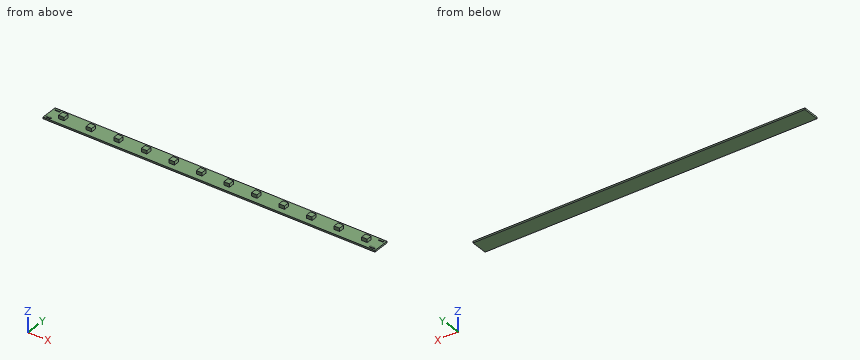
```python
from build123d import *

# Parameters (mm, degrees)
F0_W     = 200
F0_H     = 10
F1_DEPTH = 1
F2_W     = 3.3
F2_H     = 3.3
F3_DEPTH = 2
F5_DEPTH = 0.3


with BuildPart() as f1:
    # F0 (on Top) → F1 (new body)
    with BuildSketch(Plane.XY):
        with Locations((100, 5)):
            Rectangle(F0_W, F0_H)
    extrude(amount=F1_DEPTH)

    # F2 (on face) → F3 (join)
    with BuildSketch(Plane.XY.offset(1)):
        with Locations((8.65, 5)):
            Rectangle(F2_W, F2_H)
        with Locations((25.25, 5)):
            Rectangle(F2_W, F2_H)
        with Locations((41.85, 5)):
            Rectangle(F2_W, F2_H)
        with Locations((58.45, 5)):
            Rectangle(F2_W, F2_H)
        with Locations((75.05, 5)):
            Rectangle(F2_W, F2_H)
        with Locations((91.65, 5)):
            Rectangle(F2_W, F2_H)
        with Locations((108.25, 5)):
            Rectangle(F2_W, F2_H)
        with Locations((124.85, 5)):
            Rectangle(F2_W, F2_H)
        with Locations((141.45, 5)):
            Rectangle(F2_W, F2_H)
        with Locations((158.05, 5)):
            Rectangle(F2_W, F2_H)
        with Locations((174.65, 5)):
            Rectangle(F2_W, F2_H)
        with Locations((191.25, 5)):
            Rectangle(F2_W, F2_H)
    extrude(amount=F3_DEPTH)

    # F4 (on face) → F5 (join)
    with BuildSketch(Plane.XY.offset(1)):
        with BuildLine():
            ThreePointArc((1.001016, 1.177174), (1.088884, 0.965042), (1.301016, 0.877174))
            Line((1.301016, 0.877174), (3.701016, 0.877174))
            ThreePointArc((3.701016, 0.877174), (3.913148, 0.965042), (4.001016, 1.177174))
            Line((4.001016, 1.177174), (4.001016, 1.456027))
            ThreePointArc((4.001016, 1.456027), (3.913148, 1.668159), (3.701016, 1.756027))
            Line((3.701016, 1.756027), (1.301016, 1.756027))
            ThreePointArc((1.301016, 1.756027), (1.088884, 1.668159), (1.001016, 1.456027))
            Line((1.001016, 1.456027), (1.001016, 1.177174))
        make_face()
        with BuildLine():
            ThreePointArc((198.629966, 8.232874), (198.842098, 8.320742), (198.929966, 8.532874))
            Line((198.929966, 8.532874), (198.929966, 8.811727))
            ThreePointArc((198.929966, 8.811727), (198.842098, 9.023859), (198.629966, 9.111727))
            Line((198.629966, 9.111727), (196.229966, 9.111727))
            ThreePointArc((196.229966, 9.111727), (196.017834, 9.023859), (195.929966, 8.811727))
            Line((195.929966, 8.811727), (195.929966, 8.532874))
            ThreePointArc((195.929966, 8.532874), (196.017834, 8.320742), (196.229966, 8.232874))
            Line((196.229966, 8.232874), (198.629966, 8.232874))
        make_face()
        with BuildLine():
            ThreePointArc((198.629966, 0.877174), (198.842098, 0.965042), (198.929966, 1.177174))
            Line((198.929966, 1.177174), (198.929966, 1.456027))
            ThreePointArc((198.929966, 1.456027), (198.842098, 1.668159), (198.629966, 1.756027))
            Line((198.629966, 1.756027), (196.229966, 1.756027))
            ThreePointArc((196.229966, 1.756027), (196.017834, 1.668159), (195.929966, 1.456027))
            Line((195.929966, 1.456027), (195.929966, 1.277174))
            ThreePointArc((195.929966, 1.277174), (196.047123, 0.994331), (196.329966, 0.877174))
            Line((196.329966, 0.877174), (198.629966, 0.877174))
        make_face()
        with BuildLine():
            ThreePointArc((3.701016, 8.232874), (3.913148, 8.320742), (4.001016, 8.532874))
            Line((4.001016, 8.532874), (4.001016, 8.811727))
            ThreePointArc((4.001016, 8.811727), (3.913148, 9.023859), (3.701016, 9.111727))
            Line((3.701016, 9.111727), (1.301016, 9.111727))
            ThreePointArc((1.301016, 9.111727), (1.088884, 9.023859), (1.001016, 8.811727))
            Line((1.001016, 8.811727), (1.001016, 8.532874))
            ThreePointArc((1.001016, 8.532874), (1.088884, 8.320742), (1.301016, 8.232874))
            Line((1.301016, 8.232874), (3.701016, 8.232874))
        make_face()
    extrude(amount=F5_DEPTH)


solid = f1.part
```
For this review, take the finished solid that the model builds, in its own axes (mm). Coordinates: 2 decimals unless noted, no trailing zeros. Write each loop counter-clockwise with the first axis right and the second up, starting at its lowest first coordinate (ties: lowest second). Pieces come first, ordered by that corner, then holes. Notation, with made-up numbers: (15.5, 35.5) - (57.5, 35.5) arc R26 cw to (57.5, 54.5) - close; hole circle Ø10 at (-31, 66.5). An arc over 180 degrees is marked (long way). Answer in a Markdown table with one row per item. Add a question column.
Q1. We need section B-B, the plane x = 152.5. State the section outline as (y, z) points, and give its area (3 significant figures).
Q2. For P1, Ø1, axis at y = 5, z = 2, coming from the +X side; P2, Ø2, axis at x = 49.5, y = 9, coming from the +Z side; P3, Ø1, axis at x = 8.5, z = 2.5, coming from the -Y side, all flat-tipped, find the tip position at first contact; note any pin that passes through.
Q3. For probe 1 along Z at (x, y) = (161, 4.75); probe 2 along Y at (x, z) = (57.5, 2.6), list the stretches that pass through material, from the lowest coordinate up.
Q4. We need section A-A, the plane z = 2.25. Count the separate pieces of the cut face and the enclosed holes in it, and give its area (3 significant figures).
Answer list:
| question | item | result |
|---|---|---|
| 1 | outline | (0, 0) - (10, 0) - (10, 1) - (0, 1) - close |
| 1 | area | 10.0 mm2 |
| 2 | P1 | stops at x = 192.9 |
| 2 | P2 | stops at z = 1 |
| 2 | P3 | stops at y = 3.35 |
| 3 | probe 1 | z = 0 to 1 |
| 3 | probe 2 | y = 3.35 to 6.65 |
| 4 | separate pieces | 12 |
| 4 | enclosed holes | 0 |
| 4 | area | 131 mm2 |
